Design review of the part built by this model. Coordinates are the model's own, in mm. A direction names the side the tool comes from. Give positions to 0.01 mm unless a question says otherwise; leave off trailing zeros. Write each loop counter-clockwise with the first axis right and the second up, starting at its lowest first coordinate (ties: lowest second). Pieces come first, ordered by that corner, then holes. Notation, with made-up numbers: M -28,9.25 L 13,9.25 A20 ccw 13,13.25 Z; hole C 56.5,56 d7. An arc over 180 degrees is marked long. Answer in a Markdown table with one row per item.
```python
from build123d import *


with BuildPart() as f1:
    # F0 (on Front) → F1 (revolve)
    with BuildSketch(Plane.XZ):
        Polygon((-20.694755, 54.943115), (-32.936722, 54.943115), (-59.169509, 35.705738), (-30.896394, 24.629673), (-30.896394, 11.804755), (-14.282295, 11.804755), (-14.282295, -10.347377), (3.014203, -10.347377), (3.014203, 6.295834), (-4.080656, 27.25295), (51.882621, 46.198856), (47.219016, 52.31984), (10.493115, 40.952295), (8.452787, 52.31984), (-7.57836, 55.817542), (-14.573772, 48.822131), align=None)
    revolve(axis=Axis((-5.634046, 0, -10.347377), (-1, 0, 0)))


solid = f1.part
```
1) Insertion check: P1, Ø10, axis at y = 2.5, z = -8.5, coming from the +X side; P2, Ø6, axis at x = -8, y = -32.5, coming from the -Z side; P3, Ø4, axis at x = -33.5, y = -45.5, coming from the -Z side. Each pin has a flat end and moves straight along its axis. Give the tip position at first contact, or say it passes through.
Geometry says:
| item | result |
|---|---|
| P1 | x = 3.01 |
| P2 | z = -69.56 |
| P3 | z = -58.96 |
2) Add section B-B (y = 0). Write out the cut boundary in (x, z).
Geometry says:
| item | result |
|---|---|
| outline | M -59.17,-56.4 L -32.94,-75.64 L -20.69,-75.64 L -14.57,-69.52 L -7.58,-76.51 L 8.45,-73.01 L 10.49,-61.65 L 47.22,-73.01 L 51.88,-66.89 L -4.08,-47.95 L 3.01,-26.99 L 3.01,6.3 L -4.08,27.25 L 51.88,46.2 L 47.22,52.32 L 10.49,40.95 L 8.45,52.32 L -7.58,55.82 L -14.57,48.82 L -20.69,54.94 L -32.94,54.94 L -59.17,35.71 L -30.9,24.63 L -30.9,11.8 L -14.28,11.8 L -14.28,-32.5 L -30.9,-32.5 L -30.9,-45.32 Z |
3) The part is to be moulded in two halves that separate along Z. For faces 4 (the face through (11.856, -38.145, 9.493)), 5 (the face through (12.28, -50.62, -21.59)), say which applies: released by +Z, released by -Z, zero draft, split by the parting line, or undercut.
Geometry says:
| item | result |
|---|---|
| face 4 | undercut |
| face 5 | split by the parting line |
4) Add section C-C (x = -51). Write out the cut boundary in (y, z), and give its area (3 significant figures).
Geometry says:
| item | result |
|---|---|
| outline | C 0,-10.35 d104.09; hole C 0,-10.35 d85.71 |
| area | 2,740 mm^2 |
5) Add section A-A (x = 43.5). Write out the cut boundary in (y, z).
Geometry says:
| item | result |
|---|---|
| outline | C 0,-10.35 d123.03; hole C 0,-10.35 d107.42 |
6) To check wall thickness, follow probe 1 along Z at (x, y) = (-26, -18.5); probe 2 along Y at (x, z) = (25, -38.5); probe 3 along Y at (x, z) = (-53, 15.5). State the ranges of each line that lie inside material, in increasing order. Write a range as [from, to].
Geometry says:
| item | result |
|---|---|
| probe 1 | [-72.96, -22.53], [1.84, 52.27] |
| probe 2 | [-48.17, -38.19], [38.19, 48.17] |
| probe 3 | [-43.47, -35.16], [35.16, 43.47] |
7) For faces 1 (the face through (-26.9, -63.74, -24.5)), 2 (the face through (3.014, 0, -10)), 3 (the face through (-14.96, 17.89, 46.46)), list the 3-axis set-ups (+Z, -Z, +X, -X, +Y, -Y) from which the entire face can be reached by the end or side of a thin tool; tool diameter is ignored.
Geometry says:
| item | result |
|---|---|
| face 1 | -X |
| face 2 | +X |
| face 3 | none |
